```python
from build123d import *

# Parameters (mm, degrees)
SKETCH1_R                        = 48
SKETCH1_R_2                      = 8
EX_CARRIER_FRONT_PLATE_4MM_DEPTH = 2
SKETCH2_R                        = 6
CUT_PIN_HOLE_12_DEPTH            = 69
PAT_PIN_HOLES_3X120_COUNT        = 3
CUT_EXTRUDE2_DEPTH               = 1
SKETCH5_W                        = 4.5
SKETCH5_H                        = 5
SKETCH6_W                        = 10
SKETCH6_H                        = 18
BOSS_EXTRUDE1_DEPTH              = 18
SKETCH7_R                        = 2.1
CUT_EXTRUDE4_DEPTH               = 12
CIRPATTERN1_COUNT                = 3
CIRPATTERN2_COUNT                = 3


with BuildPart() as part:
    # Sketch1 → EX_Carrier_Front_Plate_4mm (new, symmetric)
    with BuildSketch(Plane.XY):
        Circle(SKETCH1_R)
        Circle(SKETCH1_R_2, mode=Mode.SUBTRACT)
    extrude(amount=EX_CARRIER_FRONT_PLATE_4MM_DEPTH, both=True)

    # Sketch2 → CUT_Pin_Hole__12 (cut, symmetric)
    with BuildSketch(Plane.XY.offset(2)):
        with Locations((0, 33.75)):
            Circle(SKETCH2_R)
    cut_pin_hole_12 = extrude(amount=CUT_PIN_HOLE_12_DEPTH, both=True, mode=Mode.SUBTRACT)

    # PAT_Pin_Holes_3x120: CUT_Pin_Hole__12 ×3 about axis
    pat_pin_holes_3x120_axis = Axis((0, 0, 0), (0, 0, 1))
    for i in range(1, PAT_PIN_HOLES_3X120_COUNT):
        add(cut_pin_hole_12.rotate(pat_pin_holes_3x120_axis, i * 360 / PAT_PIN_HOLES_3X120_COUNT), mode=Mode.SUBTRACT)

    # Sketch4 → Cut-Extrude2 (cut, symmetric)
    with BuildSketch(Plane(origin=(0, 0, 0), x_dir=(0, 0, -1), z_dir=(1, 0, 0))):
        Polygon((-2, 45.247745673), (0, 48), (-2, 48), align=None)
    extrude(amount=CUT_EXTRUDE2_DEPTH, both=True, mode=Mode.SUBTRACT)

    # Sketch5 → Revolve1 (revolve)
    with BuildSketch(Plane(origin=(0, 0, 0), x_dir=(0, 0, -1), z_dir=(1, 0, 0)), mode=Mode.PRIVATE) as revolve1_sk:
        with Locations((3.75, 10.5)):
            Rectangle(SKETCH5_W, SKETCH5_H)
    revolve(revolve1_sk.sketch.rotate(Axis((0, 0, 0), (0, 0, -1)), 90), axis=Axis((0, 0, 0), (0, 0, -1)))

    # Sketch6 → Boss-Extrude1 (add)
    with BuildSketch(Plane.XY):
        with Locations((0, -33.75)):
            Rectangle(SKETCH6_W, SKETCH6_H)
    boss_extrude1 = extrude(amount=BOSS_EXTRUDE1_DEPTH)

    # Sketch7 → Cut-Extrude4 (cut)
    with BuildSketch(Plane.XY.offset(18)):
        with Locations((0, -33.75)):
            Circle(SKETCH7_R)
    cut_extrude4 = extrude(amount=-CUT_EXTRUDE4_DEPTH, mode=Mode.SUBTRACT)

    # CirPattern1: Boss-Extrude1 ×3 about axis
    cirpattern1_axis = Axis((0, 0, 0), (0, 0, 1))
    for i in range(1, CIRPATTERN1_COUNT):
        add(boss_extrude1.rotate(cirpattern1_axis, i * 360 / CIRPATTERN1_COUNT))

    # CirPattern2: Cut-Extrude4 ×3 about axis
    cirpattern2_axis = Axis((0, 0, 0), (0, 0, 1))
    for i in range(1, CIRPATTERN2_COUNT):
        add(cut_extrude4.rotate(cirpattern2_axis, i * 360 / CIRPATTERN2_COUNT), mode=Mode.SUBTRACT)


solid = part.part
```
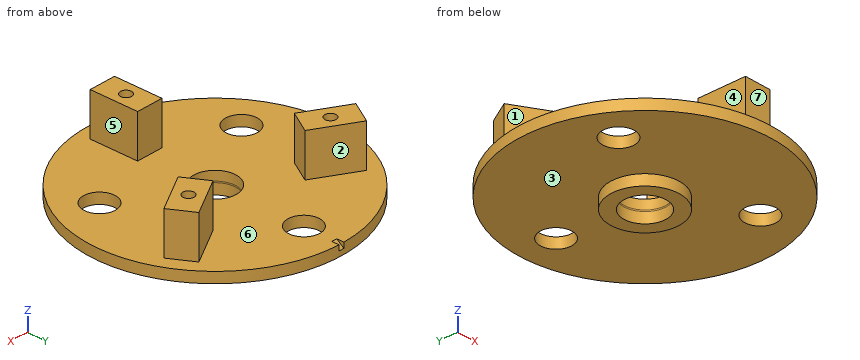
Read the model definition and answer for the solid it produces. Units are mm, in the model's axes. Face numbers are marked on the shaded views. A direction names the side the tool comes from. Coordinates: 2 decimals unless noted, no trailing zeros. Write each loop counter-clockwise with the first axis right and the second up, starting at its lowest first coordinate (ties: lowest second). Pieces come first, ordered by that corner, then holes. Notation, with made-up numbers: (-37, 61) -> (8, 61) arc R20 ccw to (8, 80) -> close; hole circle Ø11 at (-15.5, 6). An arc over 180 degrees is marked (long way). Answer as a JSON object with one key per item and string values.
Q1. The part is cut by section C-C on y = -18. Give the vertices of the cut face in (x, z).
The answers:
{"outline": "(-44.5, -2) -> (-35.12, -2) -> (-35.12, 2) -> (-44.5, 2) -> close; (-23.33, -2) -> (23.33, -2) -> (23.33, 2) -> (-23.33, 2) -> close; (35.12, -2) -> (44.5, -2) -> (44.5, 2) -> (35.12, 2) -> close"}
Q2. The part is cut by section A-A on y = 0. Give the vertices of the cut face in (x, z).
The answers:
{"outline": "(-48, -2) -> (-13, -2) -> (-13, -6) -> (-8, -6) -> (-8, 2) -> (-48, 2) -> close; (8, -6) -> (13, -6) -> (13, -2) -> (48, -2) -> (48, 2) -> (8, 2) -> close"}
Q3. The part is cut by section D-D on z = -4.5. Give the vertices of the cut face in (x, y).
The answers:
{"outline": "circle Ø26 at (0, 0); hole circle Ø16 at (0, 0)"}
Q4. Flat-ended cylindrical pins translate along their axes: pin 1 Ø8 at (x, z) = (-1.5, 9.5) entering from +Y; pin 2 Ø2 at (x, y) = (-0.5, -33.5) entering from +Z; pin 3 Ø5 at (x, y) = (-25.5, 1.5) entering from +Z; pin 4 Ø7 at (x, y) = (29.23, -16.88) entering from -Z. Find the tip coordinate at first contact, or state that the pin passes through.
The answers:
{"pin 1": "stops at y = -24.75", "pin 2": "stops at z = 6", "pin 3": "stops at z = 2", "pin 4": "passes through"}
Q5. Determine the mould class of the marked faces 4, 5, 6 and 7 for opening direction X: pulls with the +X half, pulls with the -X half, needs draft (parallel to the pull), parting line crosses it, or undercut.
The answers:
{"face 4": "pulls with the -X half", "face 5": "pulls with the +X half", "face 6": "undercut", "face 7": "needs draft"}
Q6. The part is cut by section B-B on z = 12.5. Give the vertices of the cut face in (x, y) (3 decimals).
The answers:
{"outline": "(-39.523, 17.045) -> (-23.934, 8.045) -> (-18.934, 16.705) -> (-34.523, 25.705) -> close; (-5, -42.75) -> (5, -42.75) -> (5, -24.75) -> (-5, -24.75) -> close; (18.934, 16.705) -> (23.934, 8.045) -> (39.523, 17.045) -> (34.523, 25.705) -> close; hole circle Ø4.2 at (-29.228, 16.875); hole circle Ø4.2 at (0, -33.75); hole circle Ø4.2 at (29.228, 16.875)"}
Q7. A tool of negligible diameter and unlimited length cuts with its end or side. For the marked faces 1, 2 and 3, from which of +Z, -Z, +X, -X, +Y, -Y can it reach the whole face along a straight path? Write none if from no direction.
The answers:
{"face 1": "+Z, -X, -Y", "face 2": "+Z, +Y", "face 3": "-Z"}
Q8. Consider line 1 (X direction, y = -33.5, z = 8); line 2 (Y direction, x = 0, z = -1.7); line 3 (X direction, y = 0, z = -1.75). Determine where each line is inside the solid, lowest interval first. Write a range as [from, to].
The answers:
{"line 1": "x = [-5, -2.09], [2.09, 5]", "line 2": "y = [-48, -8], [8, 27.75], [39.75, 48]", "line 3": "x = [-48, -8], [8, 48]"}
